Geometry check sheet. Reference: drawing and pictorial views, mm from the part's lowest x, y, z. A direction names the side the tool comes from. Round coordinates to 2 decimals unless told otherwise and drop trailing zeros. Order: outer loops, then holes, each group sorted by start corner. A loop starts at its lowest first (then second) coordinate and runs counter-clockwise, first axis right, second up.
(1) Sectioned sample at C-C (z = 8.75). Record the boundary of the cut face in (x, y).
(2) Release check for a two-part mould opening along X. For the marked faces 4, 5 and 6 record: +X half, -X half, draft (parallel to the pull), parting line (faces both ways), or undercut.
(3) Sectioned sample at B-B (y = 4.5). Record the boundary of the cut face in (x, z) (1 decimal).
(4) Material ranges on line 1 along Y through (x, z) = (5, 6.7); line 2 along Y through (x, z) = (5, 2.4); line 3 along X through (y, z) = (5.75, 4), recorded low to high.
(5) Sectioned sample at A-A (x = 5). Record the boundary of the cut face in (y, z).
(6) Set-up check for the marked faces 1, 2 and 3: record each of +Z, -Z, +X, -X, +Y, -Y from which the full face is reachable in a straight line by a thin tool's end or side.
(7) Go/stop test with flat-tipped pins: pin 1 (4 mm diameter, centred on x = 4.5, y = 1.5, fed in from -Z); pin 2 (1.5 mm diameter, centred on y = 8, z = 3, fed in from +X) (1 decimal); pin 3 (4 mm diameter, centred on y = 8, z = 3, fed in from -X); pin 4 (1.8 mm diameter, centred on x = 3.5, y = 5, fed in from +Z). Record where each tip stops, or that it passes through.
(8) Sectioned sample at D-D (x = 7.75). Record the boundary of the cut face in (y, z).
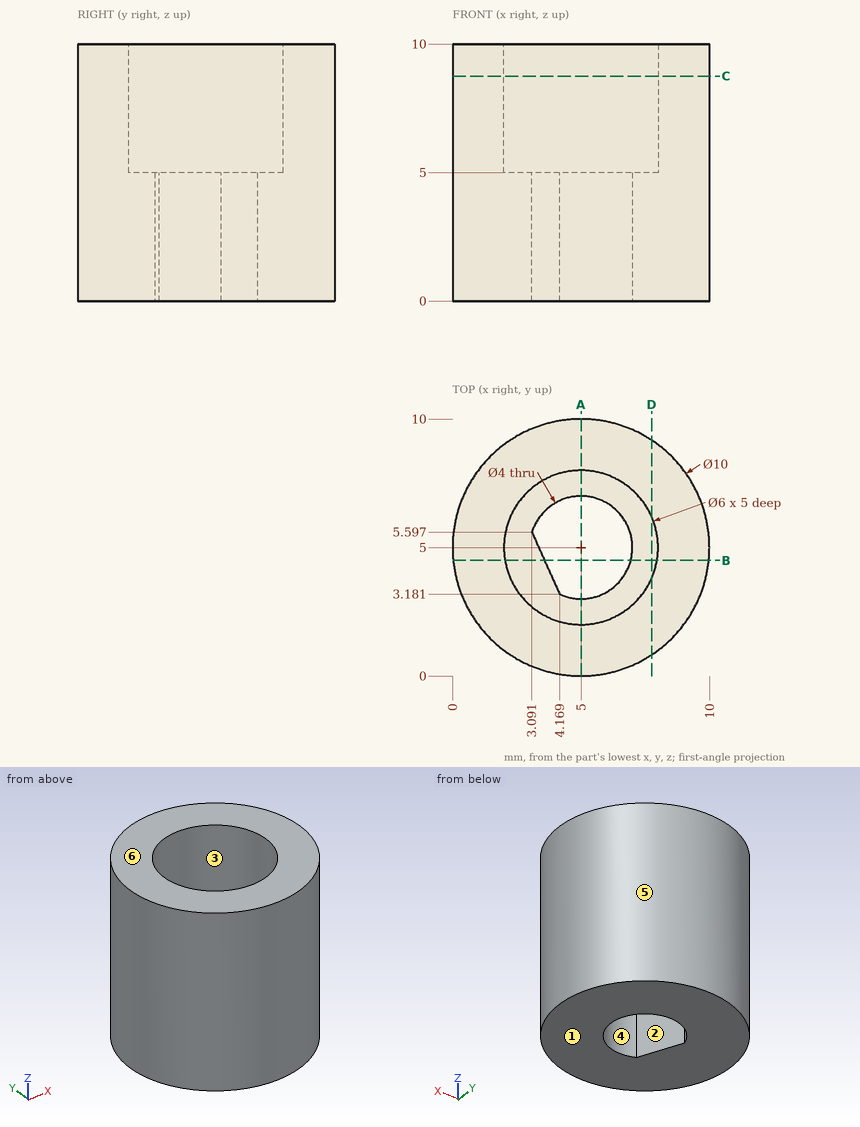
Answer below:
1. outline: circle Ø10 at (5, 5); hole circle Ø6 at (5, 5)
2. face 4: undercut
2. face 5: parting line
2. face 6: draft
3. outline: (0, 0) - (3.6, 0) - (3.6, 5) - (2, 5) - (2, 10) - (0, 10) - close; (6.9, 0) - (10, 0) - (10, 10) - (8, 10) - (8, 5) - (6.9, 5) - close
4. line 1: y = 0 to 2, 8 to 10
4. line 2: y = 0 to 3, 7 to 10
4. line 3: x = 0.06 to 3.15, 6.85 to 9.94
5. outline: (0, 0) - (3, 0) - (3, 5) - (2, 5) - (2, 10) - (0, 10) - close; (7, 0) - (10, 0) - (10, 10) - (8, 10) - (8, 5) - (7, 5) - close
6. face 1: -Z, +X, -X, +Y, -Y
6. face 2: +Z, -Z
6. face 3: +Z
7. pin 1: stops at z = 0
7. pin 2: stops at x = 9.5
7. pin 3: stops at x = 0.1
7. pin 4: stops at z = 5
8. outline: (0.82, 0) - (9.18, 0) - (9.18, 10) - (6.2, 10) - (6.2, 5) - (3.8, 5) - (3.8, 10) - (0.82, 10) - close
